Input: part model. Units: mm. Frame: model coordinates. Face numbers are marked on the shaded views. A direction names the side the tool comes from. Coordinates: 2 decimals unless noted, no trailing zeros. Write each loop counter-clockwise with the first axis right and the second up, starting at its lowest first coordinate (ties: lowest second). Pieces come first, ordered by that corner, then holes. Notation, with made-up numbers: (16.5, 77) - (66.5, 77) arc R28 cw to (66.5, 116) - close; hole circle Ø8 at (-34.5, 44). An arc over 180 degrees is marked (long way). Put each result on its own line as item: value. Start each with the question number.
1. Cut plane A-A, the plane x = 0. Return loops of the section in (y, z), and give its area (3 significant figures).
2. Pin query (flat end, axial travel): pin 1 (17 mm diameter, centred on x = 0, y = 0, fed in from -Z); pin 2 (1.5 mm diameter, centred on x = 7.5, z = 8.5, fed in from +Y); pin 3 (1 mm diameter, centred on x = 35.5, z = 8.5, fed in from -Y); pin 4 (1.5 mm diameter, centred on x = 9, z = 4.5, fed in from +Y). Return the tip coordinate at first contact, or that it passes through.
3. Pull-direction query (X, two-part tool) for the marked faces 1, 2 and 3; classes: released by +X, released by -X, zero draft, split by the parting line, or undercut.
4. Cut plane D-D, the plane x = 34.5. Return loops of the section in (y, z).
5. Line query: line 1 (Y direction, x = 0, z = 5); line 2 (X direction, y = -3, z = 7.75); line 3 (X direction, y = -5, z = 4). Output: solid intervals per line, ascending.
6. Cut plane C-C, the plane y = 3.5. Return loops of the section in (x, z).
7. Access query for the marked faces 4 and 5. Directions: +Z, -Z, +X, -X, +Y, -Y. A direction counts if a zero-diameter tool reaches every point of the face in a straight line with its end or side. Return the directions, or none.
8. Cut plane B-B, the plane z = 7.75. Return loops of the section in (x, y).
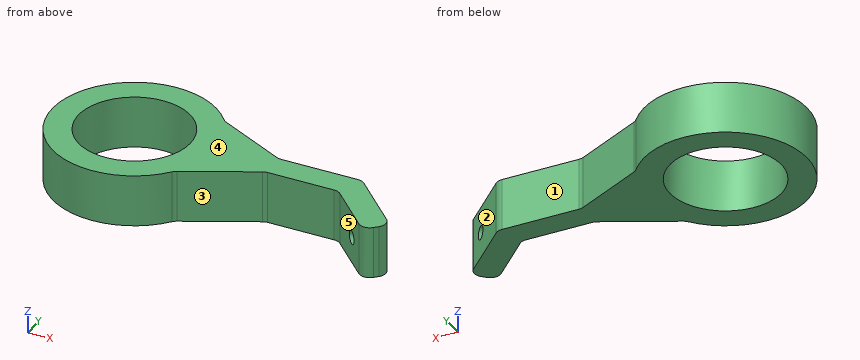
from build123d import *

# Parameters (mm, degrees)
F0_R        = 10.75
F1_DEPTH    = 10
F2_T1_DEPTH = 10
F3_R        = 1.31
F4_DEPTH    = 25
F5_R        = 2


# Not quite as in the source:
# - a fillet or chamfer that OpenCascade refuses, or shapes differently, is made with other operations: its cross-section is extruded or revolved along the edge and cut away or added


with BuildPart() as f1:
    # F0 (on Top) → F1 (new body)
    with BuildSketch(Plane.XY):
        with BuildLine():
            Line((40.75, 2.5), (15.5503215401, 2.5))
            ThreePointArc((15.5503215401, 2.5), (-15.75, 0), (15.5503215401, -2.5))
            Line((15.5503215401, -2.5), (40.75, -2.5))
            Line((40.75, -2.5), (50.295941546, -12.045941546))
            Line((50.295941546, -12.045941546), (53.831475452, -8.5104076401))
            Line((53.831475452, -8.5104076401), (42.8210678119, 2.5))
            Line((42.8210678119, 2.5), (40.75, 2.5))
        make_face()
        Circle(F0_R, mode=Mode.SUBTRACT)
    extrude(amount=F1_DEPTH)

    # F2: chamfer of 15 on 2 edges, made by hand

    # F2_s2 → F2_t1 (join)
    with BuildSketch(Plane.XY):
        with BuildLine():
            Line((27.1514391605, -2.2325951169), (12.0303066019, -9.7606848759))
            Line((12.0303066019, -9.7606848759), (11.7909271055, -9.579860495))
            ThreePointArc((11.7909271055, -9.579860495), (14.1178891417, -6.2759625701), (15.2541249393, -2.4523809524))
            Line((15.2541249393, -2.4523809524), (15.5503215401, -2.2))
            ThreePointArc((15.5503215401, -2.2), (21.3508803503, -2.2), (27.1514391605, -1.9325951169))
            Line((27.1514391605, -1.9325951169), (27.1514391605, -2.2325951169))
        make_face()
        with BuildLine():
            Line((12.0303066019, 9.7606848759), (27.1514391605, 2.2325951169))
            Line((27.1514391605, 2.2325951169), (27.1514391605, 1.9325951169))
            ThreePointArc((27.1514391605, 1.9325951169), (21.3508803503, 2.2), (15.5503215401, 2.2))
            Line((15.5503215401, 2.2), (15.2541249393, 2.4523809524))
            ThreePointArc((15.2541249393, 2.4523809524), (14.1178891417, 6.2759625701), (11.7909271055, 9.579860495))
            Line((11.7909271055, 9.579860495), (12.0303066019, 9.7606848759))
        make_face()
    extrude(amount=F2_T1_DEPTH)

    # F3 (on face) → F4 (cut)
    with BuildSketch(Plane(origin=(19.125, 19.125, 0), x_dir=(0.7071067812, -0.7071067812, 0), z_dir=(-0.7071067812, -0.7071067812, 0))):
        with Locations((38.0823682863, 5)):
            Circle(F3_R)
    extrude(amount=-F4_DEPTH, mode=Mode.SUBTRACT)

    # F5
    f5_edges = [f1.edges().sort_by_distance(p)[0] for p in [
        (50.295942, -12.045942, 5),
        (53.831475, -8.510408, 5),
        (40.75, -2.5, 5),
        (26.614322, -2.5, 5),
        (12.567424, -9.49328, 5),
        (42.821068, 2.5, 5),
        (26.614322, 2.5, 5),
        (12.567424, 9.49328, 5),
    ]]
    fillet(f5_edges, radius=F5_R)


solid = f1.part
Report:
1. outline: (-15.75, 0) - (-10.75, 0) - (-10.75, 10) - (-15.75, 10) - close; (10.75, 0) - (15.75, 0) - (15.75, 10) - (10.75, 10) - close
1. area: 100 mm^2
2. pin 1: passes through
2. pin 2: stops at y = 14.23
2. pin 3: stops at y = -2.5
2. pin 4: stops at y = 13.42
3. face 1: zero draft
3. face 2: released by +X
3. face 3: undercut
4. outline: (-2.5, 0) - (2.5, 0) - (2.5, 10) - (-2.5, 10) - close
5. line 1: y = -15.75 to -10.75, 10.75 to 15.75
5. line 2: x = -15.46 to -10.32, 10.32 to 25.61, 41.24 to 48.32
5. line 3: x = -14.94 to -9.52, 9.52 to 21.59, 43.25 to 47.66, 50.05 to 50.32
6. outline: (-15.36, 0) - (-10.16, 0) - (-10.16, 10) - (-15.36, 10) - close; (10.16, 0) - (24.61, 0) - (24.61, 10) - (10.16, 10) - close
7. face 4: +Z, +X, -X, +Y, -Y
7. face 5: +Z, -Z, -Y
8. outline: (12.3, -9.83) arc R2 cw to (12.98, -9.29) - (26.19, -2.71) arc R2 cw to (27.08, -2.5) - (39.92, -2.5) arc R2 cw to (41.34, -3.09) - (48.88, -10.63) arc R2 ccw to (51.71, -10.63) - (52.42, -9.92) arc R2 ccw to (52.42, -7.1) - (43.41, 1.91) arc R2 ccw to (41.99, 2.5) - (27.08, 2.5) arc R2 cw to (26.19, 2.71) - (12.98, 9.29) arc R2 cw to (12.3, 9.83) arc R15.75 ccw (long way) to start; hole circle Ø21.5 at (0, 0)
